The listing builds one solid part. Answer for the finished solid, in the listing's coordinates (mm). A direction names the side the tool comes from. Give positions to 0.01 mm unless a question says otherwise; leave off trailing zeros. Order: outer loops, then holes, each group sorted by start corner. A loop starts at its lowest first (then second) coordinate and runs counter-clockwise, first axis right, second up. Notation, with made-up numbers: (54, 10) -> (91, 10) arc R19 ccw to (91, 27) -> close; hole circle Ø1 at (-31, 16.25). An arc over 180 degrees is marked (long way). Answer as a JSON object with one key per item and string values. Group by question number.
```python
from build123d import *

# Parameters (mm, degrees)
SKETCH1_R           = 7.5
BOSS_EXTRUDE1_DEPTH = 54


with BuildPart() as part:
    # Sketch1 → Boss-Extrude1 (new body)
    with BuildSketch(Plane(origin=(0, 0, 0), x_dir=(1, 0, 0), z_dir=(0, 1, 0))):
        with Locations(Location((0, 0, 0), (0, 0, 270))):
            Circle(SKETCH1_R)
    extrude(amount=BOSS_EXTRUDE1_DEPTH)

    # Sketch3 → M5 Tapped Hole1 (revolve, cut)
    with BuildSketch(Plane(origin=(0, 54, 0), x_dir=(0, 0, 1), z_dir=(1, 0, 0))):
        Polygon((0, 0), (0, 13.6618073), (2.1, 12.4), (2.1, 0), align=None)
    m5_tapped_hole1 = revolve(axis=Axis((0, 60.35, 0), (0, -1, 0)), mode=Mode.SUBTRACT)

    # Mirror1: M5 Tapped Hole1 across plane
    add(m5_tapped_hole1.mirror(Plane.ZX.offset(27)), mode=Mode.SUBTRACT)


solid = part.part
```
(1) Which of the six approach directions +Z, -Z, +X, -X, +Y, -Y give full straight-line access (tool end or side, diameter ignored) to faces 4 (the cylindrical face through (-0.631, 6.113, 2.003)), 5 (the cylindrical face through (-0.631, 47.887, 2.003)), 6 (the flat face through (-2, 54, 2))?
(2) Find the intervals of material crossed by line 1 along X through (y, z) = (6.75, 0); line 2 along X through (y, z) = (10.5, 4); line 3 along X through (y, z) = (44.5, 6.5), in increasing order. Write a range as [from, to].
(3) Flat-ended cylindrical pins translate along their axes: pin 1 Ø4 at (y, z) = (28.5, 4) entering from +X; pin 2 Ø1 at (x, y) = (1.5, 15.5) entering from +Z; pin 3 Ø5 at (y, z) = (11.5, -5) entering from +X. Find the tip coordinate at first contact, or state that the pin passes through.
(4) A cutting plane is placed at B-B (z = 4.75). Determine the outline of the cut face in (x, y), and give its area (3 significant figures).
(5) A cutting plane is placed at C-C (y = 17.5). Determine the outline of the cut face in (x, z), and give its area (3 significant figures).
(6) A cutting plane is placed at D-D (z = -2.75). Determine the outline of the cut face in (x, y), and give its area (3 significant figures).
(7) For a pull along X with two mould halves and no side action, classify faces 1 (the conical face through (-0.11, 13.44, 0.35)), 2 (the flat face through (-2, 0, 2)), 3 (the cylindrical face through (0.33, 26.622, -7.493)) as +X half, -X half, draft (parallel to the pull), parting line (faces both ways), or undercut.
(8) A cutting plane is placed at A-A (y = 44). Determine the outline of the cut face in (x, z).
Check sheet entries:
{
 "1": {"face 4": "-Y", "face 5": "+Y", "face 6": "+Z, -Z, +X, -X, +Y"},
 "2": {"line 1": "x = [-7.5, -2.1], [2.1, 7.5]", "line 2": "x = [-6.34, 6.34]", "line 3": "x = [-3.74, 3.74]"},
 "3": {"pin 1": "stops at x = 7.23", "pin 2": "stops at z = 7.43", "pin 3": "stops at x = 7.07"},
 "4": {"outline": "(-5.8, 0) -> (5.8, 0) -> (5.8, 54) -> (-5.8, 54) -> close", "area": "627 mm2"},
 "5": {"outline": "circle Ø15 at (0, 0)", "area": "177 mm2"},
 "6": {"outline": "(-6.98, 0) -> (6.98, 0) -> (6.98, 54) -> (-6.98, 54) -> close", "area": "754 mm2"},
 "7": {"face 1": "undercut", "face 2": "draft", "face 3": "parting line"},
 "8": {"outline": "circle Ø15 at (0, 0); hole circle Ø4.2 at (0, 0)"}
}
